```python
from build123d import *

# Parameters (mm, degrees)
F0_R     = 8.255
F1_DEPTH = 8.89
F2_T     = -2.54
F4_DEPTH = 25.4


with BuildPart() as f1:
    # F0 (on Top) → F1 (new body)
    with BuildSketch(Plane.XY):
        with Locations((-23.585714, 0)):
            Circle(F0_R)
    extrude(amount=F1_DEPTH)

    # F2
    f2_openings = [f1.faces().sort_by_distance(p)[0] for p in [
        (-23.585714, 0, 8.89),
    ]]
    offset(amount=F2_T, openings=f2_openings)

    # F3 (on face) → F4 (cut)
    with BuildSketch(Plane(origin=(0, 0, 0), x_dir=(1, 0, 0), z_dir=(0, 0, -1))):
        with BuildLine():
            ThreePointArc((-23.191576, -0.919655), (-25.359602, -0.02163), (-24.461576, -2.189655))
            ThreePointArc((-24.461576, -2.189655), (-23.563551, -1.817681), (-23.191576, -0.919655))
        make_face()
    extrude(amount=-F4_DEPTH, mode=Mode.SUBTRACT)


solid = f1.part
```
Geometry: final body of the model. Coordinates: model frame, mm. A direction names the side the tool comes from. Coordinates: 2 decimals unless noted, no trailing zeros. Order: outer loops, then holes, each group sorted by start corner. A loop starts at its lowest first (then second) coordinate and runs counter-clockwise, first axis right, second up. Notation, with made-up numbers: (-39, -38) - (4, -38) arc R7 ccw to (4, -32) - close; hole circle Ø2 at (18, -16). An arc over 180 degrees is marked (long way). Write each question's results on one line, items separated by ' | '.
(1) First-contact query: pin 1 Ø3.5 at (x, y) = (-25, 2) entering from +Z; pin 2 Ø1.5 at (x, z) = (-25, 2) entering from +Y; pin 3 Ø1 at (y, z) = (6.5, 1) entering from +X; pin 4 Ø2 at (x, y) = (-24.46, 0.92) entering from -Z. Flat tips, straight axial feed; report the tip coordinate or a pass-through.
Values found:
pin 1: stops at z = 2.54 | pin 2: stops at y = 8.23 | pin 3: stops at x = -17.92 | pin 4: passes through
(2) Section query D-D, the plane y = -2.5. Return the cut outline in (x, z).
Values found:
outline: (-31.45, 0) - (-15.72, 0) - (-15.72, 8.89) - (-18.45, 8.89) - (-18.45, 2.54) - (-28.72, 2.54) - (-28.72, 8.89) - (-31.45, 8.89) - close
(3) Section query C-C, the plane x = -28. Return the cut outline in (y, z), plus the area to 3 significant figures.
Values found:
outline: (-6.98, 0) - (6.98, 0) - (6.98, 8.89) - (3.63, 8.89) - (3.63, 2.54) - (-3.63, 2.54) - (-3.63, 8.89) - (-6.98, 8.89) - close | area: 77.9 mm²
(4) Set-up query: faces 1 (the face through (-29.295, 0.251, 5.671)), 2 (the face through (-22, 0, 0)). Return all of +Z, -Z, +X, -X, +Y, -Y with unobstructed straight access to the full face (end or side cutting, diameter ignored); none if empty.
Values found:
face 1: +Z | face 2: -Z, +X, -X, +Y, -Y
(5) Section query B-B, the plane z = 7.75. Return the cut outline in (x, y) (3 decimals), plus the area to 3 significant figures.
Values found:
outline: circle Ø16.51 at (-23.586, 0); hole circle Ø11.43 at (-23.586, 0) | area: 111 mm²
(6) Section query A-A, the plane y = 0. Return the cut outline in (x, z), plus the area to 3 significant figures.
Values found:
outline: (-31.84, 0) - (-25.34, 0) - (-25.34, 2.54) - (-29.3, 2.54) - (-29.3, 8.89) - (-31.84, 8.89) - close; (-23.59, 0) - (-15.33, 0) - (-15.33, 8.89) - (-17.87, 8.89) - (-17.87, 2.54) - (-23.59, 2.54) - close | area: 69.7 mm²
(7) Line query: line 1 (Z direction, x = -24, y = 3.5); line 2 (Y direction, x = -23.5, z = 5); line 3 (X direction, y = -2, z = 6). Output: solid intervals per line, ascending. Write a range as [from, to].
Values found:
line 1: z = [0, 2.54] | line 2: y = [-8.25, -5.71], [5.71, 8.25] | line 3: x = [-31.59, -28.94], [-18.23, -15.58]
(8) Mould query, pull axis Y, two halves, no side actions, for faces 3 (the face through (-24, -1, 2.54)), 4 (the face through (-15.71, 2.48, 4.38)), 5 (the face through (-18, 2, 8.89)). Classes: +Y half, -Y half, draft (parallel to the pull), parting line (faces both ways), or undercut.
Values found:
face 3: undercut | face 4: parting line | face 5: draft
